from build123d import *

# Parameters (mm, degrees)
BOSS_EXTRUDE1_DEPTH     = 63.5
SKETCH5_R               = 0.55245
CUT_EXTRUDE1_DEPTH      = 64.5
CUT_EXTRUDE1_DEPTH_BACK = 64.5
SKETCH7_W               = 25.4
SKETCH7_H               = 38.1
CUT_EXTRUDE2_DEPTH      = 12.7


with BuildPart() as part:
    # Sketch4 → Boss-Extrude1 (new body, symmetric)
    with BuildSketch(Plane.XY):
        with BuildLine():
            Line((4.190365, -12.7), (10.11729625, -12.7))
            ThreePointArc((10.11729625, -12.7), (11.943543585, -11.943543585), (12.7, -10.11729625))
            Line((12.7, -10.11729625), (12.7, -4.190365))
            ThreePointArc((12.7, -4.190365), (12.42492494, -3.52627506), (11.760835, -3.2512))
            Line((11.760835, -3.2512), (11.429365, -3.2512))
            ThreePointArc((11.429365, -3.2512), (10.76527506, -3.52627506), (10.4902, -4.190365))
            Line((10.4902, -4.190365), (10.4902, -6.348478019))
            ThreePointArc((10.4902, -6.348478019), (9.830707141, -7.335478831), (8.666460301, -7.103895736))
            Line((8.666460301, -7.103895736), (5.299899128, -3.737334563))
            ThreePointArc((5.299899128, -3.737334563), (4.817571085, -3.015479634), (4.6482, -2.16399369))
            Line((4.6482, -2.16399369), (4.6482, 0))
            Line((4.6482, 0), (2.6035, 0))
            ThreePointArc((2.6035, 0), (1.840952505, -1.840952505), (0, -2.6035))
            Line((0, -2.6035), (0, -4.6482))
            Line((0, -4.6482), (2.16399369, -4.6482))
            ThreePointArc((2.16399369, -4.6482), (3.015479634, -4.817571085), (3.737334563, -5.299899128))
            Line((3.737334563, -5.299899128), (7.103895736, -8.666460301))
            ThreePointArc((7.103895736, -8.666460301), (7.335478831, -9.830707141), (6.348478019, -10.4902))
            Line((6.348478019, -10.4902), (4.190365, -10.4902))
            ThreePointArc((4.190365, -10.4902), (3.52627506, -10.76527506), (3.2512, -11.429365))
            Line((3.2512, -11.429365), (3.2512, -11.760835))
            ThreePointArc((3.2512, -11.760835), (3.52627506, -12.42492494), (4.190365, -12.7))
        make_face()
    extrude(amount=BOSS_EXTRUDE1_DEPTH, both=True)

    # Sketch5 → Cut-Extrude1 (cut, two sides)
    with BuildSketch(Plane.XY) as cut_extrude1_sk:
        with Locations((10.356153152, -12.7)):
            Circle(SKETCH5_R)
        with Locations((5.796028019, -12.7)):
            Circle(SKETCH5_R)
        with Locations((12.7, -10.356153152)):
            Circle(SKETCH5_R)
        with Locations((12.7, -5.796028019)):
            Circle(SKETCH5_R)
    extrude(amount=CUT_EXTRUDE1_DEPTH, mode=Mode.SUBTRACT)
    extrude(cut_extrude1_sk.sketch, amount=-CUT_EXTRUDE1_DEPTH_BACK, mode=Mode.SUBTRACT)

    # Mirror1: part across plane


with BuildPart() as part_1:
    add(part.part)
    add(part.part.mirror(Plane(origin=(0, 0, 0), x_dir=(0, 0, 1), z_dir=(1, 0, 0))))

    # Mirror2: part across plane


with BuildPart() as part_2:
    add(part_1.part)
    add(part_1.part.mirror(Plane.ZX))

    # Sketch7 → Cut-Extrude2 (cut, symmetric)
    with BuildSketch(Plane(origin=(0, 0, 0), x_dir=(1, 0, 0), z_dir=(0, 1, 0))):
        with Locations((0, -44.45)):
            Rectangle(SKETCH7_W, SKETCH7_H)
    extrude(amount=CUT_EXTRUDE2_DEPTH, both=True, mode=Mode.SUBTRACT)


solid = part_2.part
Read the model definition and answer for the solid it produces. Units are mm, in the model's axes. A direction names the side the tool comes from. Coordinates: 2 decimals unless noted, no trailing zeros. Answer as a JSON object with one key per item and string values.
1) The mould has two halves that part along X. Classify faces 1 (the face through (-4.648, 0, -18)), 2 (the face through (-9.847, -7.329, -18.428)), 3 (the face through (8, 12.7, -18)): released by +X, released by -X, zero draft, split by the parting line, or undercut.
Model answer:
{"face 1": "released by -X", "face 2": "undercut", "face 3": "zero draft"}
2) A tool of negligible diameter and unlimited length cuts with its end or side. For faces 4 (the face through (0, -4.648, -18)), 5 (the face through (4.822, -3.027, -18.428)), 6 (the face through (-11.931, 11.956, -18.428)), from which of +Z, -Z, +X, -X, +Y, -Y can it reach the whole face along a straight path? Write none if from no direction.
Model answer:
{"face 4": "+Z, -Z, -Y", "face 5": "+Z, -Z", "face 6": "+Z, -Z, -X, +Y"}
3) Each of these flat-tipped pins is pushed along its axis until it touches: pin 1 (2 mm diameter, centred on y = 0, z = -11, fed in from -X); pin 2 (3.5 mm diameter, centred on y = -0.5, z = -40, fed in from -X); pin 3 (1.5 mm diameter, centred on x = 7.5, y = 3, fed in from -Z); pin 4 (3.5 mm diameter, centred on y = -1, z = -38, fed in from +X). Where does it stop, or does it pass through?
Model answer:
{"pin 1": "stops at x = -4.65", "pin 2": "stops at x = -4.65", "pin 3": "passes through", "pin 4": "stops at x = 4.73"}
4) Consider line 1 along Y through (x, z) = (0, -3.5); line 2 along X through (y, z) = (4.5, -33); line 3 along X through (y, z) = (-3.5, 15). Determine where each line is inside the solid, lowest interval first. Write a range as from..to.
Model answer:
{"line 1": "y = -4.65..-2.6, 2.6..4.65", "line 2": "x = -12.7..-10.49, -6.06..6.06, 10.49..12.7", "line 3": "x = -12.4..-10.79, -5.09..5.09, 10.79..12.4"}
